Geometry: see drawing. Coordinates: mm, zero at the bounding-box minimum. Coordinates: 2 decimals unless noted, no trailing zeros. Order: outer loops, then holes, each group sorted by start corner. A loop starts at its lowest first (then second) coordinate and runs counter-clockwise, first axis right, second up. Notation, with made-up numbers: (14, 63) -> (18, 63) arc R19 ccw to (18, 86) -> close; hole circle Ø2 at (-36.75, -11.5). An arc over 180 degrees is marked (long way). One line per item, written item: value. Start each with the question number.
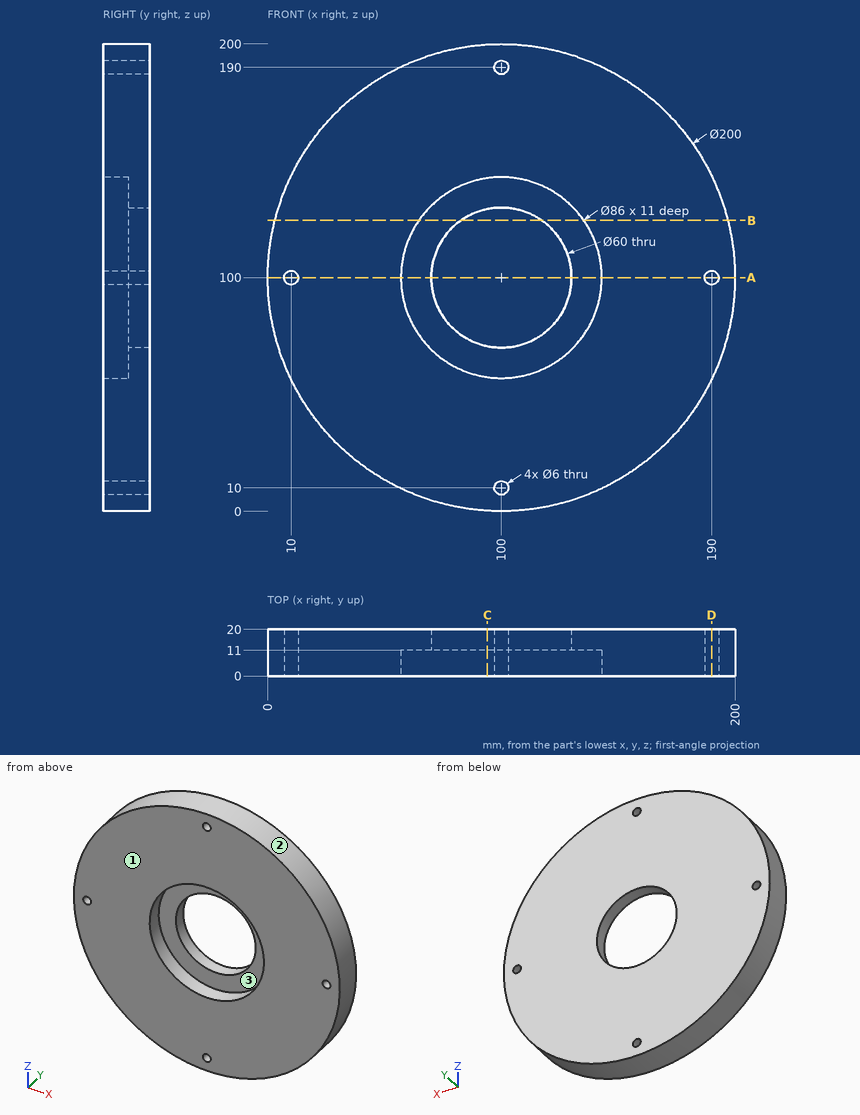
1) Section query B-B, the plane z = 124.5. Return the cut outline in (x, y).
2) Section query D-D, the plane x = 190. Return the cut outline in (y, z).
3) Mould query, pull axis X, two halves, no side actions, for the marked faces 1, 2 and 3. Classes: +X half, -X half, draft (parallel to the pull), parting line (faces both ways), or undercut.
4) Section query A-A, the plane z = 100. Return the cut outline in (x, y).
5) Section query C-C, the plane x = 94. Return the cut outline in (y, z), plus the area to 3 significant figures.
6) Ray query, line 1 along X through (y, z) = (4.25, 100); line 2 along X through (y, z) = (13, 100); line 3 along X through (y, z) = (7.5, 10). Return the intervals inside material, ascending. Write a range as from..to.
7) Pin query (flat end, axial travel): pin 1 Ø3.5 at (x, z) = (100, 10) entering from +Y; pin 2 Ø5 at (x, y) = (48, 6) entering from +Z; pin 3 Ø3 at (x, y) = (23.5, 14.5) entering from +Z; pin 4 Ø2 at (x, y) = (21.5, 10.5) entering from +Z. Return the tip coordinate at first contact, or that it passes through.
Entries:
1. outline: (3.05, 0) -> (64.66, 0) -> (64.66, 11) -> (82.69, 11) -> (82.69, 20) -> (3.05, 20) -> close; (117.31, 11) -> (135.34, 11) -> (135.34, 0) -> (196.95, 0) -> (196.95, 20) -> (117.31, 20) -> close
2. outline: (0, 56.41) -> (20, 56.41) -> (20, 97) -> (0, 97) -> close; (0, 103) -> (20, 103) -> (20, 143.59) -> (0, 143.59) -> close
3. face 1: draft
3. face 2: parting line
3. face 3: undercut
4. outline: (0, 0) -> (7, 0) -> (7, 20) -> (0, 20) -> close; (13, 0) -> (57, 0) -> (57, 11) -> (70, 11) -> (70, 20) -> (13, 20) -> close; (130, 11) -> (143, 11) -> (143, 0) -> (187, 0) -> (187, 20) -> (130, 20) -> close; (193, 0) -> (200, 0) -> (200, 20) -> (193, 20) -> close
5. outline: (0, 0.18) -> (20, 0.18) -> (20, 70.61) -> (11, 70.61) -> (11, 57.42) -> (0, 57.42) -> close; (0, 142.58) -> (11, 142.58) -> (11, 129.39) -> (20, 129.39) -> (20, 199.82) -> (0, 199.82) -> close
5. area: 2,530 mm2
6. line 1: x = 0..7, 13..57, 143..187, 193..200
6. line 2: x = 0..7, 13..70, 130..187, 193..200
6. line 3: x = 56.41..97, 103..143.59
7. pin 1: passes through
7. pin 2: stops at z = 186.89
7. pin 3: stops at z = 166.14
7. pin 4: stops at z = 163.2
